Can you work these out from the drawing? Everything is in mm from the part's minimum corner. Round coordinates to 2 decimals unless told otherwise and drop trailing zeros. Order: outer loops, then holes, each group sorted by start corner. A loop starts at its lowest first (then second) coordinate and runs counter-clockwise, first axis right, second up. Notation, with made-up numbers: (79, 50.5) -> (131, 50.5) arc R15 ccw to (131, 70.5) -> close; hole circle Ø7 at (-17, -12.5). An arc over 180 degrees is marked (long way). One line per item, written item: value.
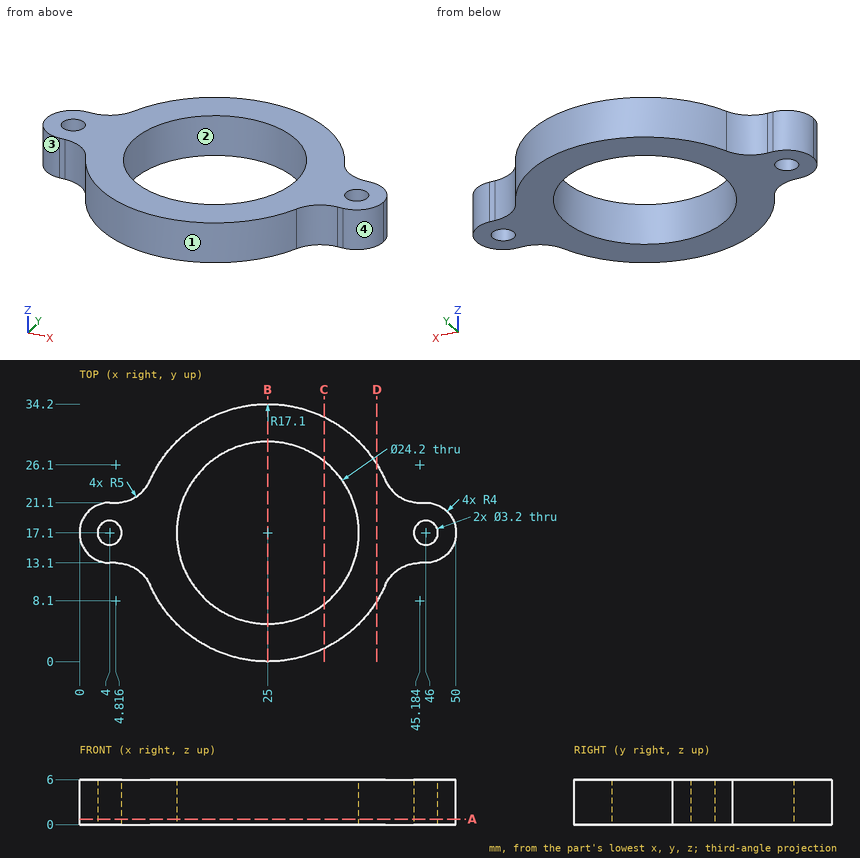
Q1. I want a section at D-D on x = 39.5. Write out the boundary of the cut face in (y, z) (1 decimal), then the cut area to 3 significant figures.
Answers:
outline: (8, 0) -> (26.2, 0) -> (26.2, 6) -> (8, 6) -> close
area: 109 mm2
Q2. I want a section at A-A on z = 0.75. Give the number of separate pieces and of enclosed holes in the cut face.
Answers:
separate pieces: 1
enclosed holes: 3
Q3. I want a section at B-B on x = 25. Write out the boundary of the cut face in (y, z), then the cut area to 3 significant figures.
Answers:
outline: (0, 0) -> (5, 0) -> (5, 6) -> (0, 6) -> close; (29.2, 0) -> (34.2, 0) -> (34.2, 6) -> (29.2, 6) -> close
area: 60.0 mm2
Q4. If we mould it in two halves opening along X, with no side actions, what happens to the marked faces 1, 2, 3 and 4? For each: pulls with the +X half, pulls with the -X half, needs draft (parallel to the pull), parting line crosses it, or undercut.
Answers:
face 1: parting line crosses it
face 2: undercut
face 3: pulls with the -X half
face 4: pulls with the +X half
Q5. I want a section at C-C on x = 32.5. Write out the boundary of the cut face in (y, z) (1 decimal).
Answers:
outline: (1.7, 0) -> (7.6, 0) -> (7.6, 6) -> (1.7, 6) -> close; (26.6, 0) -> (32.5, 0) -> (32.5, 6) -> (26.6, 6) -> close
Q6. I need wall thicknesses on line 1 along Y through (x, z) = (25, 4.7); line 2 along Y through (x, z) = (46, 3.55); line 3 along X through (y, z) = (27.5, 3.7) (1 decimal). Which ranges of each line are inside material? Lowest first, please.
Answers:
line 1: 0 to 5, 29.2 to 34.2
line 2: 13.1 to 15.5, 18.7 to 21.1
line 3: 11.4 to 18.8, 31.2 to 38.6
Q7. For P1, Ø0.7, axis at x = 45.5, z = 3, coming from the -Y side; P2, Ø19.5, axis at x = 25, y = 17.1, coming from the +Z side; P3, Ø0.9, axis at x = 4, z = 2, coming from the +Y side; P4, Ø1, axis at y = 14.5, z = 3.5, coming from the -X side (1 decimal), each with a flat end and sliding along its axis, tell me the tip position at first contact or that it passes through.
Answers:
P1: y = 13.1
P2: through
P3: y = 21.1
P4: x = 0.6
